Design review of the part shown in the three views and the two pictorial views. Dimensions are in mm from the part's minimum x, y and z. A direction names the side the tool comes from. Round coordinates to 2 decimals unless told otherwise and drop trailing zeros. Order: outer loops, then holes, each group sorted by start corner. A loop starts at its lowest first (then second) coordinate and runs counter-clockwise, first axis right, second up. Notation, with made-up numbers: M 45,27.25 L 60,27.25 A21 ccw 60,34.25 Z; hole C 74,57 d11. An arc over 180 degrees is marked long. Use a Markdown table: item, result. Add a question column.
(1) To check wall thickness, follow probe 1 along Y at (x, z) = (11.75, 7); probe 2 along X at (y, z) = (3.75, 0.5) (3 decimals); probe 3 along Z at (x, y) = (14.75, 5.25). State the ranges of each line that lie inside material, in increasing order. Write a range as from..to.
(2) For pin 1 (8 mm diameter, centred on x = 4.5, y = 18.5, fed in from -Z); pin 2 (3.5 mm diameter, centred on x = 10, z = 3, fed in from -Y); pin 3 (2.5 mm diameter, centred on x = 5.45, z = 5.6, fed in from +Y); pin 4 (2 mm diameter, centred on y = 18.5, z = 1.5, fed in from -X) (3 decimals), all flat-tipped, find the tip position at first contact; note any pin that passes through.
(3) The part is to be moulded in two halves that separate along Y. For the marked faces 4, 5 and 6, say which applies: released by +Y, released by -Y, zero draft, split by the parting line, or undercut.
(4) Machinability: for the marked faces 1, 2 and 3, which of the approach directions +Z, -Z, +X, -X, +Y, -Y give a long, thin tool a straight path to every point of the face, cutting with its end or side? Answer none if there is none.
(5) Take a section at B-B (z = 9.5). Write out the cut boundary in (x, y) (3 decimals), then the cut area to 3 significant figures.
(6) Take a section at A-A (y = 5). Write out the cut boundary in (x, z) (3 decimals).
(7) Take a section at D-D (y = 7.5). Write out the cut boundary in (x, z) (3 decimals), then the cut area to 3 significant figures.
(8) Take a section at C-C (z = 5.6). Write out the cut boundary in (x, y) (3 decimals), then the cut area to 3 significant figures.
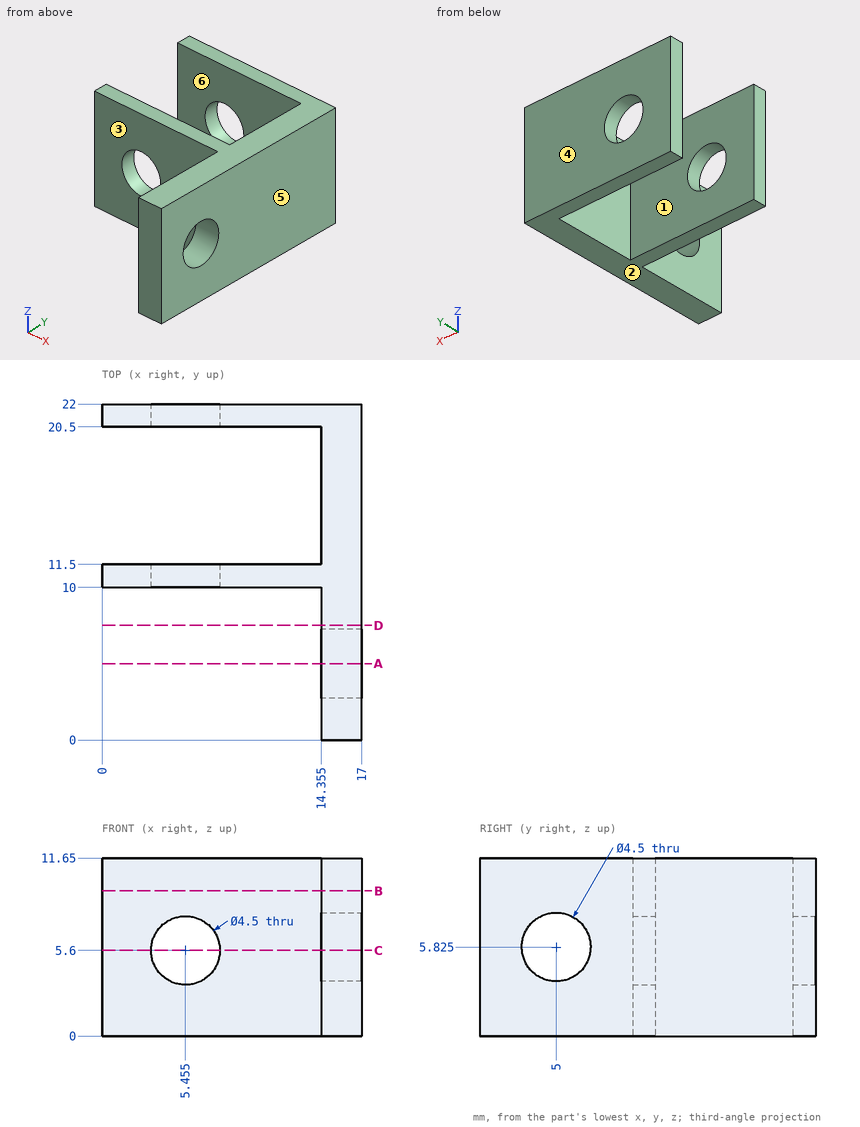
Verdict:
| question | item | result |
|---|---|---|
| 1 | probe 1 | y = 10..11.5, 20.5..22 |
| 1 | probe 2 | x = 14.355..17 |
| 1 | probe 3 | z = 0..3.59, 8.06..11.65 |
| 2 | pin 1 | stops at z = 0 |
| 2 | pin 2 | stops at y = 10 |
| 2 | pin 3 | passes through |
| 2 | pin 4 | stops at x = 14.355 |
| 3 | face 4 | released by +Y |
| 3 | face 5 | zero draft |
| 3 | face 6 | undercut |
| 4 | face 1 | +Z, -Z, -X |
| 4 | face 2 | -Z, +X, -X, +Y, -Y |
| 4 | face 3 | +Z, -Z, -X, -Y |
| 5 | outline | M 0,10 L 14.355,10 L 14.355,0 L 17,0 L 17,22 L 0,22 L 0,20.5 L 14.355,20.5 L 14.355,11.5 L 0,11.5 Z |
| 5 | area | 101 mm^2 |
| 6 | outline | M 14.355,0 L 17,0 L 17,3.575 L 14.355,3.575 Z; M 14.355,8.075 L 17,8.075 L 17,11.65 L 14.355,11.65 Z |
| 7 | outline | M 14.355,0 L 17,0 L 17,11.65 L 14.355,11.65 Z |
| 7 | area | 30.8 mm^2 |
| 8 | outline | M 0,10 L 3.205,10 L 3.205,11.5 L 0,11.5 Z; M 0,20.5 L 3.205,20.5 L 3.205,22 L 0,22 Z; M 7.705,10 L 14.355,10 L 14.355,7.239 L 17,7.239 L 17,22 L 7.705,22 L 7.705,20.5 L 14.355,20.5 L 14.355,11.5 L 7.705,11.5 Z; M 14.355,0 L 17,0 L 17,2.761 L 14.355,2.761 Z |
| 8 | area | 75.9 mm^2 |
